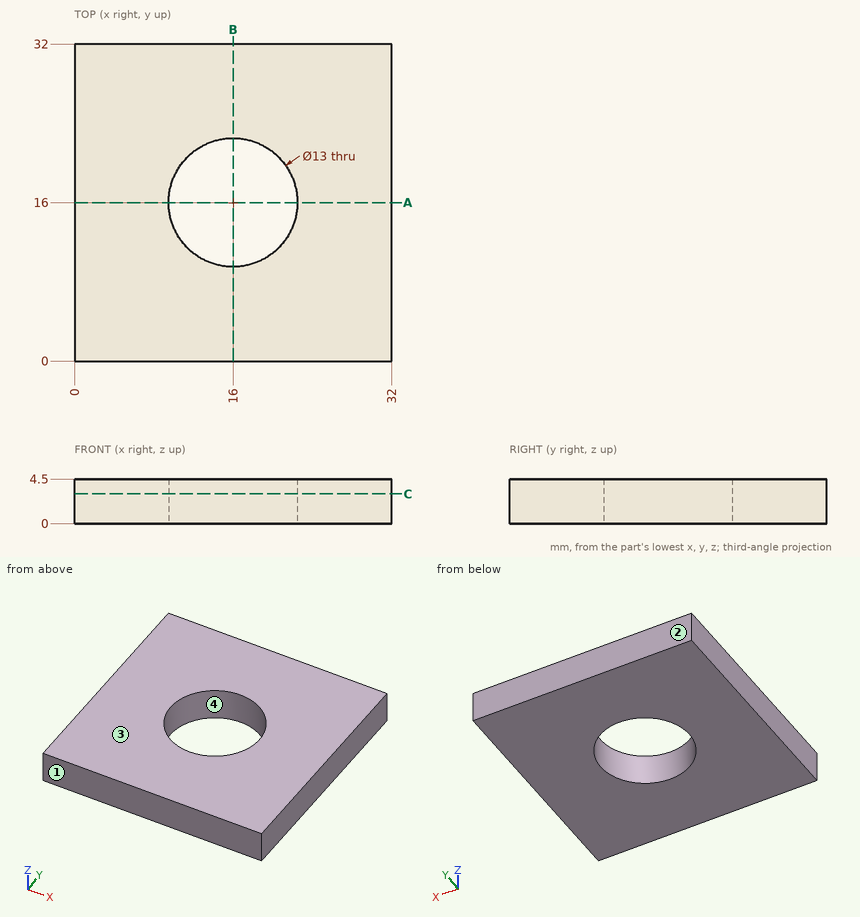
Job drawing, mm, ordinate dimensions from the low corner. One solid piece. Give positions to 0.01 mm unless a question says otherwise; leave off trailing zeros. Loops run counter-clockwise (first coordinate to the right, second up) from the corner with the lowest first, then second, coordinate; pieces in that order, holes last.
Item 1: Drill centre lines: line 1 (X direction, y = 16, z = 2.8); line 2 (X direction, y = 20, z = 2.15). Where is each one in solid material? Low to high.
Answers follow:
line 1: x = 0 to 9.5, 22.5 to 32
line 2: x = 0 to 10.88, 21.12 to 32
Item 2: Slice it at A-A, the plane y = 16. List the corners of the cut face in (x, z), and give its area (3 significant figures).
Answers follow:
outline: (0, 0) - (9.5, 0) - (9.5, 4.5) - (0, 4.5) - close; (22.5, 0) - (32, 0) - (32, 4.5) - (22.5, 4.5) - close
area: 85.5 mm2
Item 3: Pull direction Y, two halves, no side cores. Call the marked faces 1, 2, 3 and 4: released by +Y, released by -Y, zero draft, split by the parting line, or undercut.
Answers follow:
face 1: released by -Y
face 2: released by +Y
face 3: zero draft
face 4: undercut
Item 4: Slice it at C-C, the plane z = 3. List the corners of the cut face in (x, y), and give its area (3 significant figures).
Answers follow:
outline: (0, 0) - (32, 0) - (32, 32) - (0, 32) - close; hole circle Ø13 at (16, 16)
area: 891 mm2
